Geometry check sheet. Reference: the model listing, model coordinates, mm. Give positions to 0.01 mm unless a question says otherwise; leave off trailing zeros. Loops run counter-clockwise (first coordinate to the right, second up) from the corner with the lowest first, then second, coordinate; pieces in that order, holes last. Notation, with made-up numbers: (-10, 51.5) -> (35, 51.5) arc R30 ccw to (35, 73.5) -> close; hole circle Ø5 at (69.25, 72). An arc over 180 degrees is marked (long way). Write item = value, one per line. Start each with the question number.
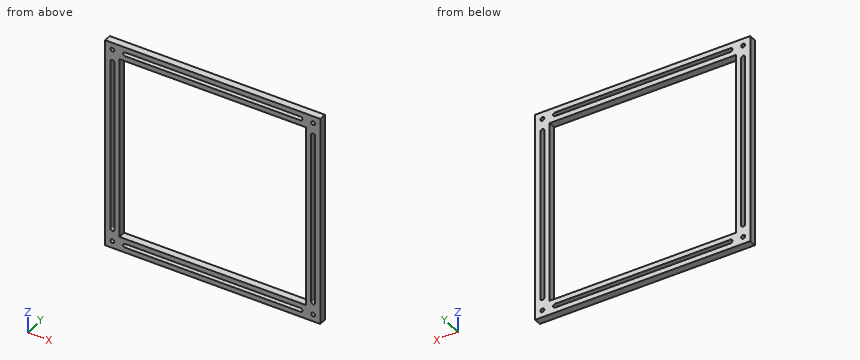
Autodesk Inventor part; units mm, degrees
ref_plane "YZ Plane" through (0, 0, 0) normal (1, 0, 0) x (0, 1, 0)
ref_plane "XZ Plane" through (0, 0, 0) normal (0, 1, 0) x (-1, 0, 0)
ref_plane "XY Plane" through (0, 0, 0) normal (0, 0, 1) x (1, 0, 0)
sketch "Sketch1" plane through (0, 0, 0) normal (0, 1, 0) x (-1, 0, 0)
  line L0 (0, 0) -> (300, 0)
  line L1 (300, 0) -> (300, -300)
  line L2 (300, -300) -> (0, -300)
  line L3 (0, -300) -> (0, 0)
  line L4 (20, -20) -> (280, -20)
  line L5 (280, -20) -> (280, -280)
  line L6 (280, -280) -> (20, -280)
  line L7 (20, -280) -> (20, -20)
  line L8 (150, 0) -> (150, -333.0511)
  line L9 (300, -150) -> (0, -150)
  line L10 (290, -23.4629) -> (290, -392.3608)
  line L11 (268.156, -10) -> (-9.9722, -10)
  line L12 (290, -27.75) -> (290, -272.25) construction
  line L13 (292.75, -27.75) -> (292.75, -272.25)
  line L14 (287.25, -272.25) -> (287.25, -27.75)
  arc A0 (292.75, -27.75) -> (287.25, -27.75) centre (290, -27.75) ccw
  arc A1 (287.25, -272.25) -> (292.75, -272.25) centre (290, -272.25) ccw
  line L15 (7.25, -27.75) -> (7.25, -272.25)
  line L16 (12.75, -272.25) -> (12.75, -27.75)
  arc A2 (12.75, -27.75) -> (7.25, -27.75) centre (10, -27.75) ccw
  arc A3 (7.25, -272.25) -> (12.75, -272.25) centre (10, -272.25) ccw
  line L17 (27.75, -10) -> (272.25, -10) construction
  line L18 (27.75, -12.75) -> (272.25, -12.75)
  line L19 (272.25, -7.25) -> (27.75, -7.25)
  arc A4 (27.75, -7.25) -> (27.75, -12.75) centre (27.75, -10) ccw
  arc A5 (272.25, -12.75) -> (272.25, -7.25) centre (272.25, -10) ccw
  line L20 (27.75, -287.25) -> (272.25, -287.25)
  line L21 (272.25, -292.75) -> (27.75, -292.75)
  arc A6 (27.75, -287.25) -> (27.75, -292.75) centre (27.75, -290) ccw
  arc A7 (272.25, -292.75) -> (272.25, -287.25) centre (272.25, -290) ccw
  line L22 (280, -280) -> (300, -300)
  circle A8 centre (290, -290) radius 2.75
  circle A9 centre (10, -290) radius 2.75
  circle A10 centre (290, -10) radius 2.75
  circle A11 centre (10, -10) radius 2.75
  point P0 (150, -20)
  point P1 (290, -150)
  point P2 (290, -25)
  point P3 (290, -275)
  point P4 (150, -10)
  point P5 (25, -10)
  point P6 (275, -10)
  point P7 (275, -290)
  dimension "d0" = 300
  dimension "d1" = 300
  dimension "d2" = 20
  dimension "d3" = 20
  dimension "d4" = 20
  dimension "d5" = 20
  dimension "d6" = 20
  dimension "d7" = 20
  dimension "d8" = 5.5
  dimension "d9" = 250
  dimension "d10" = 5.5
  dimension "d11" = 250
  dimension "d12" = 5.5
  dimension "d15" = 280
extrude "Extrusion1" add sketch "Sketch1" along normal blind 10 contours L0 L8 L19 A4 L11 A11 L3 | L0 L1 L9 L13 A0 L14 L5 L4 L8 L18 A5 L19 | L11 A11 A4 L18 L8 L4 L7 L9 L16 A2 L15 L3 | L9 L15 A3 L16 L7 L6 L8 L20 A6 L21 L2 L3 | L1 L22 A8 L10 A1 L13 L9 | L2 L10 A8 L22 | L8 L21 A7 L20 L6 L22 A8 L10 L2 | L14 A1 L10 A8 L22 L5 L9
properties part number "XYbase" material "Wood (Birch)"
1) Section check B-B (z = -95.5). Enter the section's corners in (x, y), plus the area to 3 significant figures.
2) Depth check by flat-ended pin: pin 1 Ø4.5 at (x, z) = (-10, -10) entering from -Y. Enter the tip coordinate at first touch or a pass-through.
3) Thickness scan on line 1 (X direction, y = 6.75, z = -159); line 2 (Z direction, x = -10, y = 6). Record the ranges inside material, lowest first.
4) Section check C-C (y = 5.5). Give the number of separate pieces and of enclosed holes in the cut face, plus the area to 3 significant figures.
5) Section check A-A (x = -142.5). Enter the section's corners in (y, z), plus the area to 3 significant figures.
Check result:
q1.outline = (-300, 0) -> (-292.75, 0) -> (-292.75, 10) -> (-300, 10) -> close; (-287.25, 0) -> (-280, 0) -> (-280, 10) -> (-287.25, 10) -> close; (-20, 0) -> (-12.75, 0) -> (-12.75, 10) -> (-20, 10) -> close; (-7.25, 0) -> (0, 0) -> (0, 10) -> (-7.25, 10) -> close
q1.area = 290 mm2
q2.pin_1 = through
q3.line_1 = -300 to -292.75, -287.25 to -280, -20 to -12.75, -7.25 to 0
q3.line_2 = -300 to -292.75, -287.25 to -275, -25 to -12.75, -7.25 to 0
q4.separate_pieces = 1
q4.enclosed_holes = 9
q4.area = 16,800 mm2
q5.outline = (0, -300) -> (10, -300) -> (10, -292.75) -> (0, -292.75) -> close; (0, -287.25) -> (10, -287.25) -> (10, -280) -> (0, -280) -> close; (0, -20) -> (10, -20) -> (10, -12.75) -> (0, -12.75) -> close; (0, -7.25) -> (10, -7.25) -> (10, 0) -> (0, 0) -> close
q5.area = 290 mm2
